```python
from build123d import *

# Parameters (mm, degrees)
F0_W     = 65
F0_H     = 12
F1_DEPTH = 5
F3_DEPTH = 65.001
F4_W     = 6
F4_H     = 12
F5_DEPTH = 3


with BuildPart() as f1:
    # F0 (on Front) → F1 (new body)
    with BuildSketch(Plane.XZ):
        Rectangle(F0_W, F0_H)
    extrude(amount=-F1_DEPTH)

    # F2 (on face) → F3 (cut, through all)
    with BuildSketch(Plane(origin=(-32.5, 0, 0), x_dir=(0, -1, 0), z_dir=(-1, 0, 0))):
        Polygon((0, -6), (0, -1), (-5, -6), align=None)
    extrude(amount=-F3_DEPTH, mode=Mode.SUBTRACT)

    # F4 (on face) → F5 (cut)
    with BuildSketch(Plane.XZ):
        with Locations((29.5, 0)):
            Rectangle(F4_W, F4_H)
        with Locations((-29.5, 0)):
            Rectangle(F4_W, F4_H)
    extrude(amount=-F5_DEPTH, mode=Mode.SUBTRACT)


solid = f1.part
```
Here's how the part is built. I have some questions about the finished solid (model axes, mm). A direction names the side the tool comes from. Coordinates: 2 decimals unless noted, no trailing zeros. Order: outer loops, then holes, each group sorted by start corner. A loop starts at its lowest first (then second) coordinate and runs counter-clockwise, first axis right, second up. Notation, with made-up numbers: (25.25, 12.25) - (34.25, 12.25) arc R9 ccw to (34.25, 28.25) - close; hole circle Ø2 at (53, 62). An arc over 180 degrees is marked (long way). One line per question, with ' | ' between items.
(1) If I drill on L1, parallel to X at y = 2.1, z = -0.75; L2, parallel to Y at x = 28, z = 5.25; L3, parallel to Z at x = -4, y = 3, over which ranges is the centre line in solid material (lowest first)?
Report:
L1: x = -26.5 to 26.5 | L2: y = 3 to 5 | L3: z = -4 to 6
(2) Will these pins go through, and if not, where does the flat tip stop? pin 1 (3 mm diameter, centred on x = -17.5, z = 3, fed in from -Y); pin 2 (3 mm diameter, centred on y = 0.5, z = -0.5, fed in from -X); pin 3 (1.8 mm diameter, centred on x = -30.5, z = 2.5, fed in from -Y); pin 4 (0.9 mm diameter, centred on y = 1.5, z = 3.5, fed in from +X).
Report:
pin 1: stops at y = 0 | pin 2: stops at x = -26.5 | pin 3: stops at y = 3 | pin 4: stops at x = 26.5
(3) Suppose I cut it at A-A on z = 0.5. List the corners of the cut face in (x, y) for me, and give its area (3 significant figures).
Report:
outline: (-32.5, 3) - (-26.5, 3) - (-26.5, 0) - (26.5, 0) - (26.5, 3) - (32.5, 3) - (32.5, 5) - (-32.5, 5) - close | area: 289 mm2
(4) For faces 1 (the flat face through (29, 3, 1)), 2 (the flat face through (-32.5, 4, 0)), 3 (the flat face through (-30, 3, 1)), which set-ups out of +Z, -Z, +X, -X, +Y, -Y let a thin tool reach every point of the face, with its end or its side?
Report:
face 1: +Z, -Z, +X, -Y | face 2: +Z, -Z, -X, +Y, -Y | face 3: +Z, -Z, -X, -Y
(5) Suppose I cut it at B-B on y = 0.8. List the corners of the cut face in (x, z) for me.
Report:
outline: (-26.5, -1.8) - (26.5, -1.8) - (26.5, 6) - (-26.5, 6) - close
(6) Suppose I cut it at C-C on x = 9. List the corners of the cut face in (y, z) for me, and give its area (3 significant figures).
Report:
outline: (0, -1) - (5, -6) - (5, 6) - (0, 6) - close | area: 47.5 mm2
